Design review of the part built by this model. Coordinates are the model's own, in mm. A direction names the side the tool comes from. Coordinates: 2 decimals unless noted, no trailing zeros. Loops run counter-clockwise (first coordinate to the right, second up) from the corner with the lowest first, then second, coordinate; pieces in that order, holes last. Notation, with made-up numbers: M 23,-30 L 48,-30 A16 ccw 48,-19 Z; hole C 3.5,1.25 d6. An arc over 180 degrees is marked long. Put each result on its own line as item: value. Start each with the question number.
(1) Clearance check with flat-ended pins moving along their axes: pin 1 (1 mm diameter, centred on x = -8.5, z = 0.5, fed in from +Y); pin 2 (8 mm diameter, centred on x = -11.5, z = 22.5, fed in from -Y); pin 3 (5 mm diameter, centred on y = 99.5, z = 26, fed in from +X). State where each tip first meets the part, or that it passes through.
(2) For faces 4 (the flat face through (-8.03, 91.34, 10.02)), 5 (the flat face through (-4.592, 83.043, -1.565)), 6 (the flat face through (-24.686, 131.555, -1.565)), list the 3-axis set-ups (+Z, -Z, +X, -X, +Y, -Y) from which the entire face can be reached by the end or side of a thin tool; tool diameter is ignored.
(3) For probe 1 along Z at (x, y) = (-15, 116); probe 2 along Z at (x, y) = (-5, 89.5) (3 decimals); probe 3 along X at (y, z) = (82, 2), list the stretches that pass through material, from the lowest coordinate up. Write a range as [from, to].
(4) Take a section at B-B, the plane z = 5. Give the boundary of the cut face in (x, y).
(5) Take a section at A-A, the plane z = -1. Give the boundary of the cut face in (x, y).
(6) The part is to be moulded in two halves that separate along Y. For faces 1 (the flat face through (-27.198, 137.387, -1.565)), 2 (the flat face through (-24, 130, 0)), 3 (the flat face through (-4, 81, 0)), say which applies: +Y half, -Y half, draft (parallel to the pull), parting line (faces both ways), or undercut.
(7) Take a section at C-C, the plane z = 9. Give the boundary of the cut face in (x, y).
(8) Take a section at D-D, the plane x = 1.5. Give the boundary of the cut face in (y, z) (3 decimals), then the cut area to 3 significant figures.
Autodesk Inventor part; units mm, degrees
ref_plane "YZ Plane" through (0, 0, 0) normal (1, 0, 0) x (0, 1, 0)
ref_plane "XZ Plane" through (0, 0, 0) normal (0, 1, 0) x (-1, 0, 0)
ref_plane "XY Plane" through (0, 0, 0) normal (0, 0, 1) x (1, 0, 0)
ref_plane "Work Plane1" through (0, 0, 0) normal (0, 0, 1) x (1, 0, 0)
sketch "Sketch1" plane through (0, 0, 0) normal (0, 0, 1) x (1, 0, 0)
  line L0 (0, 152.4) -> (-45.5982, 133.5126)
  line L1 (-31.4153, 139.3873) -> (-25.5487, 141.8174)
  line L2 (-25.5487, 141.8174) -> (3.6118, 71.4178)
  line L3 (3.6118, 71.4178) -> (-2.2548, 68.9877)
  line L4 (-2.2548, 68.9877) -> (-31.4153, 139.3873)
  point P0 (0, 0)
  dimension "d0" = 6.35
  dimension "d1" = 76.2
extrude "Extrusion1" add sketch "Sketch1" along normal blind 31.75
sketch "Sketch2" plane through (-25.5487, 141.8174, 31.75) normal (0.9238795, 0.3826834, 0) x (0, 0, -1)
  line L0 (11.43, -52.324) -> (11.43, -13.716)
  line L1 (30.734, -53.34) -> (12.446, -53.34)
  line L2 (12.446, -12.7) -> (20.955, -12.7)
  line L3 (11.43, -53.34) -> (11.43, -12.7)
  line L4 (11.43, -12.7) -> (31.75, -12.7)
  line L5 (31.75, -12.7) -> (31.75, -53.34)
  line L6 (31.75, -53.34) -> (11.43, -53.34)
  point P0 (31.75, -140.7992)
extrude "Extrusion2" cut sketch "Sketch2" against normal through all
sketch "Sketch3" plane through (-25.5487, 141.8174, 31.75) normal (0.9238795, 0.3826834, 0) x (0, 0, -1)
  arc A0 (18.161, -58.6942) -> (14.859, -58.6942) centre (16.51, -57.15) ccw
  arc A1 (28.321, -58.6942) -> (25.019, -58.6942) centre (26.67, -57.15) ccw
  arc A2 (14.859, -7.3458) -> (18.161, -7.3458) centre (16.51, -8.89) ccw
  arc A3 (25.019, -7.3458) -> (28.321, -7.3458) centre (26.67, -8.89) ccw
  circle A4 centre (16.51, -57.15) radius 2.2606
  circle A5 centre (26.67, -57.15) radius 2.2606
  circle A6 centre (16.51, -8.89) radius 2.2606
  circle A7 centre (26.67, -8.89) radius 2.2606
  point P0 (31.75, -140.7992)
extrude "Extrusion3" cut sketch "Sketch3" against normal through all
sketch "Sketch4" plane through (0, 0, 0) normal (0, 0, -1) x (-1, 0, 0)
  line L0 (11.003, 90.1076) -> (5.1363, 92.5377) construction
  line L1 (5.1363, 92.5377) -> (-3.6118, 71.4178) construction
  line L2 (-3.6118, 71.4178) -> (2.2548, 68.9877) construction
  line L3 (2.2548, 68.9877) -> (11.003, 90.1076) construction
  line L4 (20.6886, 130.0841) -> (26.5552, 127.6541) construction
  line L5 (26.5552, 127.6541) -> (31.4153, 139.3873) construction
  line L6 (31.4153, 139.3873) -> (25.5487, 141.8174) construction
  line L7 (25.5487, 141.8174) -> (20.6886, 130.0841) construction
  line L8 (24.224, 138.6194) -> (21.794, 132.7528)
  line L9 (21.794, 132.7528) -> (27.6606, 130.3227)
  line L10 (27.6606, 130.3227) -> (30.0907, 136.1894)
  line L11 (30.0907, 136.1894) -> (24.224, 138.6194)
  line L12 (4.1298, 90.1076) -> (1.6998, 84.241)
  line L13 (1.6998, 84.241) -> (7.5664, 81.8109)
  line L14 (7.5664, 81.8109) -> (9.9964, 87.6776)
  line L15 (9.9964, 87.6776) -> (4.1298, 90.1076)
  line L16 (-0.2443, 79.5477) -> (-2.6743, 73.681)
  line L17 (-2.6743, 73.681) -> (3.1923, 71.251)
  line L18 (3.1923, 71.251) -> (5.6224, 77.1176)
  line L19 (5.6224, 77.1176) -> (-0.2443, 79.5477)
  point P0 (0, 0)
  dimension "d8" = 6.35
  dimension "d9" = 6.35
  dimension "d10" = 6.35
  dimension "d11" = 6.35
  dimension "d12" = 6.35
extrude "Extrusion4" add sketch "Sketch4" along normal blind 3.175
properties part number "servoMountPlate"
Computed values:
1. pin 1: stops at y = 91.35
1. pin 2: stops at y = 81.65
1. pin 3: stops at x = -6.98
2. face 4: -Z, -X, +Y
2. face 5: -Z, +X
2. face 6: -Z, +X, -Y
3. probe 1: z = [20.32, 31.75]
3. probe 2: z = [-3.175, 3.029], [7.131, 13.189], [17.291, 31.75]
3. probe 3: x = [-7.64, -0.77]
4. outline: M -31.42,139.39 L -28.88,133.26 L -23.01,135.69 L -25.55,141.82 Z; M -27.15,129.09 L -26.56,127.65 L -20.69,130.08 L -21.28,131.52 Z; M -11,90.11 L -10.41,88.67 L -4.54,91.1 L -5.14,92.54 Z; M -8.68,84.5 L -2.25,68.99 L 3.61,71.42 L -2.81,86.93 Z
5. outline: M -30.09,136.19 L -27.66,130.32 L -21.79,132.75 L -24.22,138.62 Z; M -10,87.68 L -7.57,81.81 L -1.7,84.24 L -4.13,90.11 Z; M -5.62,77.12 L -3.19,71.25 L 2.67,73.68 L 0.24,79.55 Z
6. face 1: +Y half
6. face 2: draft
6. face 3: undercut
7. outline: M -31.42,139.39 L -26.56,127.65 L -20.69,130.08 L -25.55,141.82 Z; M -11,90.11 L -2.25,68.99 L 3.61,71.42 L -5.14,92.54 Z
8. outline: M 70.543,0 L 73.195,0 L 73.195,-3.175 L 76.516,-3.175 L 76.516,31.75 L 70.543,31.75 Z
8. area: 200 mm^2
